from build123d import *

# Parameters (mm, degrees)
SKETCH1_W           = 288.925
SKETCH1_H           = 247.65
SKETCH1_W_2         = 273.05
SKETCH1_H_2         = 231.775
BOSS_EXTRUDE1_DEPTH = 20.6375
SKETCH2_W           = 231.775
SKETCH2_H           = 2.839616755
BOSS_EXTRUDE2_DEPTH = 273.05
SKETCH3_R           = 2.54
CUT_EXTRUDE1_DEPTH  = 356.620697252


with BuildPart() as part:
    # Sketch1 → Boss-Extrude1 (new body)
    with BuildSketch(Plane(origin=(0, 0, 0), x_dir=(1, 0, 0), z_dir=(0, 1, 0))):
        with Locations((47.164436759, -82.481854668)):
            Rectangle(SKETCH1_W, SKETCH1_H)
        with Locations((47.164436759, -82.481854668)):
            Rectangle(SKETCH1_W_2, SKETCH1_H_2, mode=Mode.SUBTRACT)
    extrude(amount=BOSS_EXTRUDE1_DEPTH)

    # Sketch2 → Boss-Extrude2 (add)
    with BuildSketch(Plane(origin=(-89.360563241, 0, 0), x_dir=(0, 0, -1), z_dir=(1, 0, 0))):
        with Locations((-82.481854668, 1.419808378)):
            Rectangle(SKETCH2_W, SKETCH2_H)
    extrude(amount=BOSS_EXTRUDE2_DEPTH)

    # Sketch3 → Cut-Extrude1 (cut, through all)
    with BuildSketch(Plane(origin=(191.626936759, 0, 0), x_dir=(0, 0, -1), z_dir=(1, 0, 0))):
        with Locations((-82.481854668, 10.31875)):
            Circle(SKETCH3_R)
    extrude(amount=-CUT_EXTRUDE1_DEPTH, mode=Mode.SUBTRACT)


solid = part.part
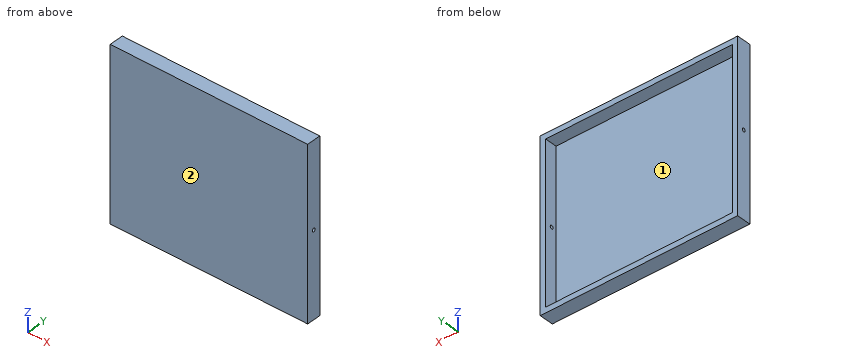
The model under review builds one solid part; all positions refer to its coordinate system, in mm. Face numbers are marked on the shaded views. Round coordinates to 2 decimals unless told otherwise and drop trailing zeros. Write each loop counter-clockwise with the first axis right and the second up, starting at its lowest first coordinate (ties: lowest second). Pieces come first, ordered by that corner, then holes. Notation, with made-up numbers: (86.25, 53.5) -> (127.25, 53.5) arc R25 ccw to (127.25, 82.5) -> close; hole circle Ø7 at (72, 62). An arc over 180 degrees is marked (long way). Answer as a JSON object with one key per item and string values.
1. We need section C-C on z = 43.5. State the section outline as (x, y) points, and give its area (3 significant figures).
Results found:
{"outline": "(-97.3, 0) -> (191.63, 0) -> (191.63, 20.64) -> (183.69, 20.64) -> (183.69, 2.84) -> (-89.36, 2.84) -> (-89.36, 20.64) -> (-97.3, 20.64) -> close", "area": "1,100 mm^2"}
2. We need section A-A on y = 16. State the section outline as (x, z) points, and give its area (3 significant figures).
Results found:
{"outline": "(-97.3, -41.34) -> (191.63, -41.34) -> (191.63, 206.31) -> (-97.3, 206.31) -> close; hole (-89.36, -33.41) -> (183.69, -33.41) -> (183.69, 198.37) -> (-89.36, 198.37) -> close", "area": "8,270 mm^2"}
3. The part is to be moulded in two halves that separate along X. For the marked faces 1 and 2, say which applies: pulls with the +X half, pulls with the -X half, needs draft (parallel to the pull), parting line crosses it, or undercut.
Results found:
{"face 1": "undercut", "face 2": "needs draft"}
4. We need section B-B on x = 46. State the section outline as (y, z) points.
Results found:
{"outline": "(0, -41.34) -> (20.64, -41.34) -> (20.64, -33.41) -> (2.84, -33.41) -> (2.84, 198.37) -> (20.64, 198.37) -> (20.64, 206.31) -> (0, 206.31) -> close"}
5. To check wall thickness, follow line 1 along X through (y, z) = (18.75, 35.5); line 2 along Z through (x, y) = (31, 6.25); line 3 along Y through (x, z) = (78.5, 20.5). State the ranges of each line that lie inside material, in increasing order.
Results found:
{"line 1": "x = -97.3 to -89.36, 183.69 to 191.63", "line 2": "z = -41.34 to -33.41, 198.37 to 206.31", "line 3": "y = 0 to 2.84"}
6. Clearance check with flat-ended pins moving along their axes: pin 1 (3 mm diameter, centred on x = 88.5, z = 132.5, fed in from +Y); pin 2 (6.5 mm diameter, centred on y = 10.32, z = 82.48, fed in from -X). State where each tip first meets the part, or that it passes through.
Results found:
{"pin 1": "stops at y = 2.84", "pin 2": "stops at x = -97.3"}
